Part model, mm, in its own coordinate system. Face numbers are marked on the shaded views. A direction names the side the tool comes from. Give positions to 0.01 mm unless a question says otherwise; leave off trailing zeros. Loops run counter-clockwise (first coordinate to the right, second up) from the corner with the lowest first, then second, coordinate; pieces in that order, holes last. Notation, with made-up numbers: (48, 60.5) -> (62, 60.5) arc R31 ccw to (62, 95.5) -> close; hole circle Ø1 at (79.5, -4.75). An arc over 180 degrees is marked (long way). Write item = value, one per line.
from build123d import *

# Parameters (mm, degrees)
SKETCH_2_OUTSIDE_W  = 33.106
SKETCH_2_OUTSIDE_H  = 33.106
CUT_EXTRUDE_1_DEPTH = 64.42710304
CHAMFER_1_SIZE      = 1


with BuildPart() as part:
    # Эскиз1 → Повернуть1 (revolve)
    with BuildSketch(Plane.XY, mode=Mode.PRIVATE) as revolve_1_sk:
        Polygon((-6.58, 0), (-6.58, 8.85), (0, 8.85), (0, 7.448974596), (0.6, 7.288205081), (0.6, 5), (55.6, 5), (55.6, 0), align=None)
    revolve(revolve_1_sk.sketch.rotate(Axis((-1000, 0, 0), (1, 0, 0)), 90), axis=Axis((-1000, 0, 0), (1, 0, 0)))

    # Эскиз2 outside → Вырез-Вытянуть1 (cut, through all)
    with BuildSketch(Plane.ZY.offset(6.58)):
        Rectangle(SKETCH_2_OUTSIDE_W, SKETCH_2_OUTSIDE_H)
        Polygon((0, -8.85), (7.664324823, -4.425), (7.664324823, 4.425), (0, 8.85), (-7.664324823, 4.425), (-7.664324823, -4.425), align=None, mode=Mode.SUBTRACT)
    extrude(amount=-CUT_EXTRUDE_1_DEPTH, mode=Mode.SUBTRACT)

    # Эскиз4 → Вырез-Повернуть1 (revolve, cut)
    with BuildSketch(Plane.XY):
        Polygon((-6.58, 8.075), (-6.297923068, 8.85), (-6.58, 8.85), align=None)
    revolve(axis=Axis((-1000, 0, 0), (1, 0, 0)), mode=Mode.SUBTRACT)

    # Фаска1
    chamfer_1_edges = [part.edges().sort_by_distance(p)[0] for p in [
        (55.6, 0, -5),
    ]]
    chamfer(chamfer_1_edges, length=CHAMFER_1_SIZE)


solid = part.part
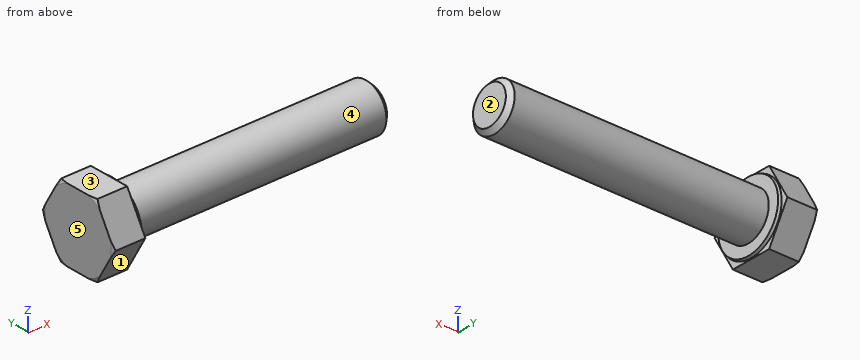
1) Drop flat-ended pins along their axis: P1, Ø10, axis at x = 36.5, y = -3.5, coming from the -Z side; P2, Ø3, axis at x = 27.5, y = -0.5, coming from the +Z side; P3, Ø1.5, axis at x = 30, y = 6.5, coming from the -Z side; P4, Ø6, axis at x = 23, z = -2, coming from the -Y side. Give the stop position or say it passes through.
Resolved:
P1 = -5
P2 = 5
P3 = through
P4 = -5
2) Slice it at B-B, the plane x = 5. List the corners of the cut face in (y, z), and give its area (3 significant figures).
Resolved:
outline = circle Ø10 at (0, 0)
area = 78.5 mm²
3) Which spindle directions (+Z, -Z, +X, -X, +Y, -Y) get a long thin tool onto all of the face, cutting with end or side? Do the marked faces 4 and 5. Say none if no direction does.
Resolved:
face_4 = +X
face_5 = +Z, -Z, -X, +Y, -Y
4) Drill centre lines: line 1 along X through (y, z) = (-4.75, -3.5); line 2 along Z through (x, y) = (23.5, -4); line 3 along Z through (x, y) = (1, -4.5). Where is each one in solid material? Low to high. Write a range as [from, to].
Resolved:
line_1 = [-6.58, 0.6]
line_2 = [-3, 3]
line_3 = [-2.18, 2.18]
5) Pull direction Z, two halves, no side cores. Call the marked faces 1, 2 and 3: pulls with the +Z half, pulls with the -Z half, needs draft (parallel to the pull), parting line crosses it, or undercut.
Resolved:
face_1 = pulls with the -Z half
face_2 = needs draft
face_3 = pulls with the +Z half
6) Slice it at A-A, the plane y = 0. List the corners of the cut face in (x, z), and give its area (3 significant figures).
Resolved:
outline = (-6.58, -7.66) -> (0, -7.66) -> (0, -7.45) -> (0.6, -7.29) -> (0.6, -5) -> (54.6, -5) -> (55.6, -4) -> (55.6, 4) -> (54.6, 5) -> (0.6, 5) -> (0.6, 7.29) -> (0, 7.45) -> (0, 7.66) -> (-6.58, 7.66) -> close
area = 659 mm²
